Geometry: final body of the model. Coordinates: model frame, mm. Face numbers are marked on the shaded views. A direction names the side the tool comes from. Round coordinates to 2 decimals unless told otherwise and drop trailing zeros. Loops run counter-clockwise (first coordinate to the right, second up) from the corner with the lowest first, then second, coordinate; pieces in that order, holes last. Notation, with made-up numbers: (71.5, 84) - (115.5, 84) arc R28 cw to (115.5, 122) - close; hole circle Ø5 at (-12.75, 1). An arc over 180 degrees is marked (long way). Answer in a Markdown table with one row per item. Add a question column.
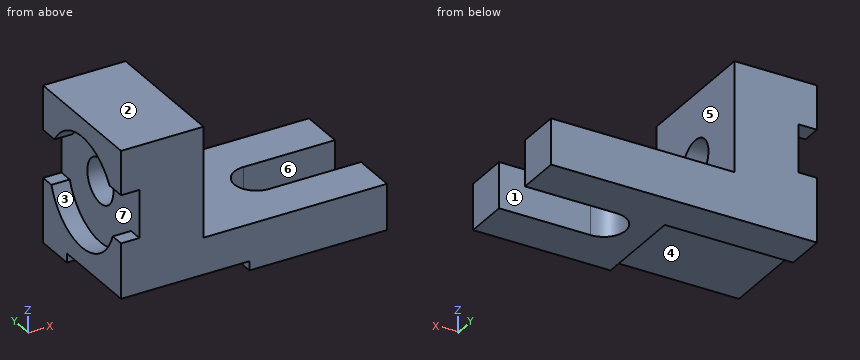
from build123d import *

# Parameters (mm, degrees)
SKETCH1_W           = 135
SKETCH1_H           = 72
BOSS_EXTRUDE2_DEPTH = 25
SKETCH2_W           = 60
SKETCH2_H           = 5
CUT_EXTRUDE1_DEPTH  = 72
CUT_EXTRUDE2_DEPTH  = 153
SKETCH4_W           = 30
SKETCH4_H           = 72
BOSS_EXTRUDE3_DEPTH = 10
SKETCH7_W           = 5
SKETCH7_H           = 22
BOSS_EXTRUDE4_DEPTH = 70
SKETCH9_W           = 35
SKETCH9_H           = 72
BOSS_EXTRUDE5_DEPTH = 60
SKETCH10_W          = 10
SKETCH10_H          = 24
BOSS_EXTRUDE6_DEPTH = 72
CUT_EXTRUDE3_DEPTH  = 10
SKETCH12_R          = 12
CUT_EXTRUDE4_DEPTH  = 42


with BuildPart() as part:
    # Sketch1 → Boss-Extrude2 (new body)
    with BuildSketch(Plane.XY):
        with Locations((67.5, -36)):
            Rectangle(SKETCH1_W, SKETCH1_H)
    extrude(amount=BOSS_EXTRUDE2_DEPTH)

    # Sketch2 → Cut-Extrude1 (cut)
    with BuildSketch(Plane.XZ.offset(72)):
        with Locations((30, 2.5)):
            Rectangle(SKETCH2_W, SKETCH2_H)
    extrude(amount=-CUT_EXTRUDE1_DEPTH, mode=Mode.SUBTRACT)

    # Sketch3 → Cut-Extrude2 (cut)
    with BuildSketch(Plane.XY):
        with BuildLine():
            Line((135, -24), (85, -24))
            ThreePointArc((85, -24), (73, -36), (85, -48))
            Line((85, -48), (135, -48))
            Line((135, -48), (135, -24))
        make_face()
    extrude(amount=CUT_EXTRUDE2_DEPTH, mode=Mode.SUBTRACT)

    # Sketch4 → Boss-Extrude3 (add)
    with BuildSketch(Plane.ZY):
        with Locations((20, -36)):
            Rectangle(SKETCH4_W, SKETCH4_H)
    extrude(amount=BOSS_EXTRUDE3_DEPTH)

    # Sketch7 → Boss-Extrude4 (add)
    with BuildSketch(Plane.ZY.offset(10)):
        with Locations((2.5, -11)):
            Rectangle(SKETCH7_W, SKETCH7_H)
    extrude(amount=-BOSS_EXTRUDE4_DEPTH)

    # Sketch9 → Boss-Extrude5 (add)
    with BuildSketch(Plane.XY.offset(25)):
        with Locations((17.5, -36)):
            Rectangle(SKETCH9_W, SKETCH9_H)
    extrude(amount=BOSS_EXTRUDE5_DEPTH)

    # Sketch10 → Boss-Extrude6 (add)
    with BuildSketch(Plane.XZ.offset(72)):
        with Locations((-5, 73)):
            Rectangle(SKETCH10_W, SKETCH10_H)
    extrude(amount=-BOSS_EXTRUDE6_DEPTH)

    # Sketch11 → Cut-Extrude3 (cut)
    with BuildSketch(Plane.ZY.offset(10)):
        with BuildLine():
            Line((35, -7.715728753), (35, -64.284271247))
            ThreePointArc((35, -64.284271247), (15, -36), (35, -7.715728753))
        make_face()
        with BuildLine():
            Line((61, -10.622844919), (61, -61.377155081))
            ThreePointArc((61, -61.377155081), (75, -36), (61, -10.622844919))
        make_face()
    extrude(amount=-CUT_EXTRUDE3_DEPTH, mode=Mode.SUBTRACT)

    # Sketch12 → Cut-Extrude4 (cut)
    with BuildSketch(Plane.ZY):
        with Locations((48, -36)):
            Circle(SKETCH12_R)
    extrude(amount=-CUT_EXTRUDE4_DEPTH, mode=Mode.SUBTRACT)


solid = part.part
1) Reachability of the marked faces 4, 5, 6 and 7 from +Z, -Z, +X, -X, +Y, -Y: full face, straight path, thin tool, end or side. Return the list, or none.
2) Material intervals for line 1 along Y through (x, z) = (14, 48); line 2 along X through (y, z) = (-6, 76); line 3 along Z through (x, y) = (92.5, -52), sorted ascending. Write a range as from..to.
3) Section A-A, the plane x = 117.5. Return the cut outline in (y, z), and give its area (3 significant figures).
4) Section C-C, the plane x = 17.5. Return the cut outline in (y, z).
5) Pull-direction query (Z, two-part tool) for the marked faces 1, 2 and 3; classes: pulls with the +Z half, pulls with the -Z half, needs draft (parallel to the pull), parting line crosses it, or undercut.
6) Section D-D, the plane y = -36. Return the cut outline in (x, z), and give its area (4 significant figures).
7) Section B-B, the plane z = 48. Return the cut outline in (x, y).
8) Contact query for flat-ended pins moving along their axis: pin 1 Ø2.5 at (y, z) = (-43.5, 1.5) entering from -X; pin 2 Ø1.5 at (x, z) = (16.5, 1.5) entering from -Y; pin 3 Ø1 at (y, z) = (-38, 14.5) entering from +X; pin 4 Ø14.5 at (y, z) = (-36, 48) entering from +X. Output: stop coordinate, or through.
Evaluation:
| question | item | result |
|---|---|---|
| 1 | face 4 | -Z, -X, -Y |
| 1 | face 5 | +Z, +X, +Y, -Y |
| 1 | face 6 | +Z, -Z, +X |
| 1 | face 7 | -X |
| 2 | line 1 | y = -72..-48, -24..0 |
| 2 | line 2 | x = -10..35 |
| 2 | line 3 | z = 0..25 |
| 3 | outline | (-72, 0) - (-48, 0) - (-48, 25) - (-72, 25) - close; (-24, 0) - (0, 0) - (0, 25) - (-24, 25) - close |
| 3 | area | 1,200 mm² |
| 4 | outline | (-72, 5) - (-22, 5) - (-22, 0) - (0, 0) - (0, 85) - (-72, 85) - close; hole circle Ø24 at (-36, 48) |
| 5 | face 1 | needs draft |
| 5 | face 2 | pulls with the +Z half |
| 5 | face 3 | undercut |
| 6 | outline | (-10, 5) - (60, 5) - (60, 0) - (73, 0) - (73, 25) - (35, 25) - (35, 36) - (0, 36) - (0, 15) - (-10, 15) - close; (-10, 75) - (0, 75) - (0, 60) - (35, 60) - (35, 85) - (-10, 85) - close |
| 6 | area | 2,985 mm² |
| 7 | outline | (0, -72) - (35, -72) - (35, -48) - (0, -48) - close; (0, -24) - (35, -24) - (35, 0) - (0, 0) - close |
| 8 | pin 1 | stops at x = 60 |
| 8 | pin 2 | stops at y = -22 |
| 8 | pin 3 | stops at x = 73.26 |
| 8 | pin 4 | passes through |
